```python
from build123d import *
from build123d.topology import SkipClean

# Parameters (mm, degrees)
ESQUISSE1_W             = 100
ESQUISSE1_H             = 100
ESQUISSE1_R             = 2.75
BOSS_EXTRU_1_DEPTH      = 5
BOSS_EXTRU_2_START      = 29
ESQUISSE2_R             = 2.75
BOSS_EXTRU_2_DEPTH      = 29
ESQUISSE3_W             = 30
ESQUISSE3_H             = 43.5
BOSS_EXTRU_3_DEPTH      = 29
CHANFREIN1_SIZE         = 29
CHANFREIN1_SIZE_2       = 45.5
ENL_V_START             = -30
ESQUISSE4_R             = 2.75
ENL_V_MAT_EXTRU_1_DEPTH = 30
ESQUISSE7_W             = 10
ESQUISSE7_H             = 29
ENL_V_MAT_EXTRU_2_DEPTH = 77.426435217


with BuildPart() as part:
    # Esquisse1 → Boss.-Extru.1 (new body)
    with BuildSketch(Plane(origin=(0, 0, 0), x_dir=(1, 0, 0), z_dir=(0, 1, 0))):
        Rectangle(ESQUISSE1_W, ESQUISSE1_H)
        with Locations(Location((0, -15, 0), (0, 0, 270))):
            Circle(ESQUISSE1_R, mode=Mode.SUBTRACT)
    extrude(amount=BOSS_EXTRU_1_DEPTH)

    # Esquisse2 → Boss.-Extru.2 (add)
    with SkipClean():  # the faces are left unmerged after this step: merging them gives an invalid solid
        with BuildSketch(Plane.XZ.offset(BOSS_EXTRU_2_START)):
            with BuildLine():
                ThreePointArc((-15, 15), (0, 30), (15, 15))
                Line((15, 15), (15, -1.5))
                Line((15, -1.5), (-15, -1.5))
                Line((-15, -1.5), (-15, 15))
            make_face()
            with Locations(Location((0, 15, 0), (0, 0, 270))):
                Circle(ESQUISSE2_R, mode=Mode.SUBTRACT)
        extrude(amount=-BOSS_EXTRU_2_DEPTH)

    # Esquisse3 → Boss.-Extru.3 (add)
    with SkipClean():  # the faces are left unmerged after this step: merging them gives an invalid solid
        with BuildSketch(Plane.XZ):
            with Locations((0, -23.25)):
                Rectangle(ESQUISSE3_W, ESQUISSE3_H)
        extrude(amount=BOSS_EXTRU_3_DEPTH)

    # Chanfrein1
    # the kernel refuses this chamfer: 45.5, 29 mm, written as the material it takes off along each edge
    with BuildSketch(Plane(origin=(-132.612350115, -29, -45), x_dir=(0, 0.9986920470194074, -0.051129201247289646), z_dir=(1, 0, 0))) as chanfrein1_piece_1_section:
        Polygon((CHANFREIN1_SIZE * 0.998692047019, CHANFREIN1_SIZE * 0.0511292012473), (-CHANFREIN1_SIZE_2 * 0.0511292012473, CHANFREIN1_SIZE_2 * 0.998692047019), (0, 0), align=None)
    chanfrein1_piece_1 = extrude(amount=265.22470023, mode=Mode.PRIVATE)
    chanfrein1_piece_1 = split(chanfrein1_piece_1, bisect_by=Plane(origin=(0, 0, -29.75832693), z_dir=(0, -1, 0)), keep=Keep.TOP, mode=Mode.PRIVATE)
    add(chanfrein1_piece_1, mode=Mode.SUBTRACT)

    # Esquisse4 → Enlèv. mat.-Extru.1 (cut)
    with BuildSketch(Plane(origin=(0, 5, 0), x_dir=(1, 0, 0), z_dir=(0, 1, 0)).offset(ENL_V_START)):
        Polygon((4.05, -17.33826859), (4.05, -12.66173141), (0, -10.32346282), (-4.05, -12.66173141), (-4.05, -17.33826859), (0, -19.67653718), align=None)
        with Locations(Location((0, -15, 0), (0, 0, 90))):
            Circle(ESQUISSE4_R, mode=Mode.SUBTRACT)
    extrude(amount=ENL_V_MAT_EXTRU_1_DEPTH, mode=Mode.SUBTRACT)

    # Esquisse7 → Enlèv. mat.-Extru.2 (cut, through all)
    with BuildSketch(Plane.XY):
        with Locations((-5, -14.5)):
            Rectangle(ESQUISSE7_W, ESQUISSE7_H)
        with Locations((5, -14.5)):
            Rectangle(ESQUISSE7_W, ESQUISSE7_H)
    extrude(amount=-ENL_V_MAT_EXTRU_2_DEPTH, mode=Mode.SUBTRACT)


solid = part.part
```
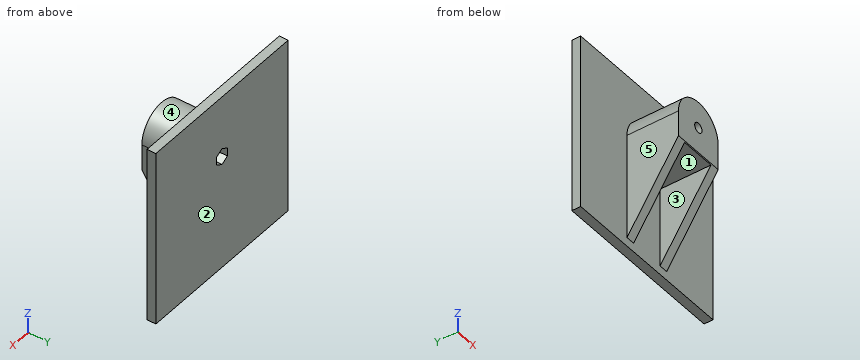
The listing builds one solid part. Answer for the finished solid, in the listing's coordinates (mm). Face numbers are marked on the shaded views. A direction names the side the tool comes from. Coordinates: 2 decimals unless noted, no trailing zeros. Write each loop counter-clockwise with the first axis right and the second up, starting at its lowest first coordinate (ties: lowest second). Pieces come first, ordered by that corner, then holes. Notation, with made-up numbers: (85, 33.25) -> (121, 33.25) arc R18 ccw to (121, 39.25) -> close; hole circle Ø1 at (67.5, 16.25). An arc over 180 degrees is marked (long way). Write each question's results on one line, items separated by ' | '. Start each with the question number.
1) Straight lines are drawn through the part: probe 1 along Z at (x, y) = (0, -26); probe 2 along X at (y, z) = (-27, 15); probe 3 along X at (y, z) = (-9, -13). For each, find the intervals that lie inside material, in ascending order.
2) A cutting plane is placed at D-D (x = 27). Determine the outline of the cut face in (y, z), then the cut area to 3 significant figures.
3) For a pull along X with two mould halves and no side action, classify the marked faces 3, 4 and 5 as +X half, -X half, draft (parallel to the pull), parting line (faces both ways), or undercut.
4) A cutting plane is placed at C-C (x = -13). Determine the outline of the cut face in (y, z).
5) A cutting plane is placed at B-B (y = -17.5). Determine the outline of the cut face in (x, z).
6) A cutting plane is placed at A-A (z = 3). Determine the outline of the cut face in (x, y).
7) A tool of negligible diameter and unlimited length cuts with its end or side. For the marked faces 1 and 2, from which of +Z, -Z, +X, -X, +Y, -Y can it reach the whole face along a straight path? Write none if from no direction.
8) Flat-ended cylindrical pins translate along their axes: pin 1 Ø12 at (y, z) = (-8.5, 24) entering from -X; pin 2 Ø8.5 at (y, z) = (-18, -23) entering from +X; pin 3 Ø3 at (y, z) = (-11.5, -28.5) entering from -X. Find the tip coordinate at first contact, or state that the pin passes through.
Values follow:
1) probe 1: 0 to 12.25, 17.75 to 30 | probe 2: -15 to -2.75, 2.75 to 15 | probe 3: -15 to -10, 10 to 15
2) outline: (0, -50) -> (5, -50) -> (5, 50) -> (0, 50) -> close | area: 500 mm²
3) face 3: undercut | face 4: parting line | face 5: -X half
4) outline: (-29, 0.5) -> (0, -45) -> (0, -50) -> (5, -50) -> (5, 50) -> (0, 50) -> (0, 22.48) -> (-29, 22.48) -> close
5) outline: (-15, -17.54) -> (-10, -17.54) -> (-10, 0) -> (10, 0) -> (10, -17.54) -> (15, -17.54) -> (15, 15) arc R15 ccw to (-15, 15) -> close; hole (-4.05, 12.66) -> (0, 10.32) -> (4.05, 12.66) -> (4.05, 17.34) -> (0, 19.68) -> (-4.05, 17.34) -> close
6) outline: (-50, 0) -> (-15, 0) -> (-15, -29) -> (15, -29) -> (15, 0) -> (50, 0) -> (50, 5) -> (-50, 5) -> close
7) face 1: -Z, -Y | face 2: +Z, -Z, +X, -X, +Y
8) pin 1: x = -14.7 | pin 2: x = 15 | pin 3: x = -15
